from build123d import *

# Parameters (mm, degrees)
SKETCH1_R              = 1.95
SKETCH1_R_2            = 2.2
MAIN_BODY_DEPTH        = 6.91
SKETCH2_R              = 1
TENDON_HOLE_DEPTH      = 10
MATERIAL_REMOVAL_DEPTH = 5


with BuildPart() as part:
    # Sketch1 → main body (new body)
    with BuildSketch(Plane.XY):
        with BuildLine():
            Line((-17.760263169, -1), (-2.775337817, -1))
            ThreePointArc((-2.775337817, -1), (2.95, 0), (-2.775337817, 1))
            Line((-2.775337817, 1), (-17.760263169, 1))
            ThreePointArc((-17.760263169, 1), (-24, 0), (-17.760263169, -1))
        make_face()
        Circle(SKETCH1_R, mode=Mode.SUBTRACT)
        with Locations((-20.8, 0)):
            Circle(SKETCH1_R_2, mode=Mode.SUBTRACT)
    extrude(amount=MAIN_BODY_DEPTH)

    # Sketch2 → tendon hole (cut, symmetric)
    with BuildSketch(Plane.XZ.offset(1)):
        with Locations((-20.840065792, 3.455)):
            Circle(SKETCH2_R)
    extrude(amount=TENDON_HOLE_DEPTH, both=True, mode=Mode.SUBTRACT)

    # Sketch3 → material removal (cut, symmetric)
    with BuildSketch(Plane.XZ.offset(1)):
        with BuildLine():
            Line((-2.775337817, 3.455), (2.95, 3.455))
            Line((2.95, 3.455), (2.95, 0))
            Line((2.95, 0), (-2.775337817, 0))
            Line((-2.775337817, 0), (-17.760263169, 0))
            ThreePointArc((-17.760263169, 0), (-10.464372425, 2.580066057), (-2.775337817, 3.455))
        make_face()
    extrude(amount=MATERIAL_REMOVAL_DEPTH, both=True, mode=Mode.SUBTRACT)


solid = part.part
Check sheet for the modelled part. Datum: model origin and axes. Units: mm. A direction names the side the tool comes from. Coordinates: 2 decimals unless noted, no trailing zeros. Write each loop counter-clockwise with the first axis right and the second up, starting at its lowest first coordinate (ties: lowest second). Pieces come first, ordered by that corner, then holes.
Item 1: Cross-section at C-C on z = 5.5. Record the boundary of the cut face in (x, y).
Numbers:
outline: (-17.76, -1) - (-2.78, -1) arc R2.95 ccw (long way) to (-2.78, 1) - (-17.76, 1) arc R3.2 ccw (long way) to start; hole circle Ø4.4 at (-20.8, 0); hole circle Ø3.9 at (0, 0)
Item 2: Cross-section at B-B on y = 0. Record the boundary of the cut face in (x, z) (3 decimals), then the cut area to 3 significant figures.
Numbers:
outline: (-24, 0) - (-23, 0) - (-23, 6.91) - (-24, 6.91) - close; (-18.6, 0) - (-17.76, 0) arc R34.224 cw to (-2.775, 3.455) - (-1.95, 3.455) - (-1.95, 6.91) - (-18.6, 6.91) - close; (1.95, 3.455) - (2.95, 3.455) - (2.95, 6.91) - (1.95, 6.91) - close
area: 87.7 mm2
Item 3: Cross-section at D-D on z = 1.25. Record the boundary of the cut face in (x, y), then the cut area to 3 significant figures.
Numbers:
outline: (-17.76, -1) - (-14.86, -1) - (-14.86, 1) - (-17.76, 1) arc R3.2 ccw (long way) to start; hole circle Ø4.4 at (-20.8, 0)
area: 22.5 mm2
Item 4: Access from +Z, -Z, +X, -X, +Y, -Y to the whole of each face (thin tool, end or side, straight path). Record for faces 1 (the face through (-12, 1, 4)), 2 (the face through (-12, -1, 4)), 3 (the face through (-19.9, -2.6, 3.8)), 4 (the face through (2, 1, 3.455)).
Numbers:
face 1: +Z, -Z, +Y
face 2: +Z, -Z, -Y
face 3: +Y, -Y
face 4: -Z, +X, +Y, -Y
Item 5: Scan lines: probe 1 along Y at (x, z) = (0, 5.8); probe 2 along Y at (x, z) = (-20.8, 4.5); probe 3 along X at (y, z) = (2, 6). Record each from-to range of solid material in increasing order.
Numbers:
probe 1: y = -2.95 to -1.95, 1.95 to 2.95
probe 2: y = -3.2 to -2.2, 2.2 to 3.2
probe 3: x = -23.3 to -21.72, -19.88 to -18.3, -2.17 to 2.17
Item 6: Cross-section at A-A on x = 0. Record the boundary of the cut face in (y, z) (3 decimals).
Numbers:
outline: (-2.95, 3.455) - (-1.95, 3.455) - (-1.95, 6.91) - (-2.95, 6.91) - close; (1.95, 3.455) - (2.95, 3.455) - (2.95, 6.91) - (1.95, 6.91) - close
Item 7: Mould release check, pull along X, two halves, no side actions. Record for faces 5 (the face through (-11, 0, 6.91)), 6 (the face through (-10.57, -0.014, 2.556)), 7 (the face through (-18.768, -0.843, 3.407)): released by +X, released by -X, zero draft, split by the parting line, or undercut.
Numbers:
face 5: zero draft
face 6: released by +X
face 7: undercut
Item 8: Depth check by flat-ended pin: pin 1 Ø1.5 at (y, z) = (-1.5, 3.5) entering from +X; pin 2 Ø3 at (y, z) = (-1.5, 2) entering from -X; pin 3 Ø2 at (x, z) = (-9.5, 2) entering from +Y. Enter the tip coordinate at first touch or a pass-through.
Numbers:
pin 1: stops at x = 2.85
pin 2: stops at x = -24
pin 3: stops at y = 1
